Model file for the job. Use its own axes, mm. A direction names the side the tool comes from. Coordinates: 2 decimals unless noted, no trailing zeros. Order: outer loops, then holes, each group sorted by start corner. A loop starts at its lowest first (then second) coordinate and runs counter-clockwise, first axis right, second up. Notation, with made-up numbers: (-39, 80) -> (-12, 80) arc R30 cw to (-12, 119) -> close; hole circle Ø1 at (17.25, -19.75). An arc over 180 degrees is marked (long way). Return JSON: item names as keys, results as strings. Group by question number.
1) Cut at C-C (y = 46.5). Write the cut outline in (x, z), and give its area (3 significant figures).
2) Which spindle directions (+Z, -Z, +X, -X, +Y, -Y) get a long thin tool onto all of the face, cutting with end or side? Do faces 1 (the flat face through (15, 7, 13)), 2 (the flat face through (0, 35, 0)), 3 (the flat face through (11, 38, 0)), 4 (the flat face through (12.4, 10, -0.3)). Say none if no direction does.
3) Cut at D-D (y = 4). Write the cut outline in (x, z).
4) Pull direction Z, two halves, no side cores. Call faces 5 (the flat face through (-9, 7, -19)), 6 (the flat face through (-19, 5, 0)), 7 (the cylindrical face through (-8.895, 8.521, -17.615)), 8 (the cylindrical face through (-11.99, 25.84, -0.53)): +Z half, -Z half, draft (parallel to the pull), parting line (faces both ways), or undercut.
5) Cut at A-A (z = -16). Write the cut outline in (x, y).
6) Flat gauge pins, fed straight in: pin 1 (7 mm diameter, centred on y = 40, z = -2, fed in from +X); pin 2 (14 mm diameter, centred on x = -12, z = -16, fed in from +Y); pin 3 (19 mm diameter, centred on x = 12, z = 16, fed in from -Y); pin 4 (2 mm diameter, centred on y = 18, z = -10.5, fed in from +X). Where does each tip first touch, or does it go through?
7) Cut at B-B (z = 16). Write the cut outline in (x, y), and give its area (3 significant figures).
8) Probe line 1 (Z direction, x = -12, y = 8); line 2 (X direction, y = 6, z = 16); line 3 (Z direction, x = -12, y = 4.5). List the from-to ranges inside material, lowest first.
Autodesk Inventor part; units mm, degrees
ref_plane "YZ Plane" through (0, 0, 0) normal (1, 0, 0) x (0, 1, 0)
ref_plane "XZ Plane" through (0, 0, 0) normal (0, 1, 0) x (-1, 0, 0)
ref_plane "XY Plane" through (0, 0, 0) normal (0, 0, 1) x (1, 0, 0)
sketch "Эскиз1" plane through (0, 0, 0) normal (0, 0, 1) x (1, 0, 0)
  line L0 (-19, 10) -> (19, 10)
  line L1 (19, 10) -> (19, 0)
  line L2 (19, 0) -> (-19, 0)
  line L3 (-19, 0) -> (-19, 10)
  line L4 (12, 10) -> (12, 34)
  line L5 (12, 34) -> (11, 34)
  line L6 (11, 34) -> (11, 50)
  line L7 (11, 50) -> (4, 50)
  line L8 (4, 50) -> (4, 35)
  line L9 (4, 35) -> (0, 35)
  line L10 (0, 35) -> (0, 10)
  line L11 (12, 34) -> (12, 50)
  line L12 (12, 50) -> (11, 50)
  line L13 (4, 50) -> (-4, 50)
  line L14 (-4, 50) -> (-4, 35)
  line L15 (-4, 35) -> (0, 35)
  line L16 (-12, 34) -> (-11, 34)
  line L17 (-11, 34) -> (-11, 50)
  line L18 (-12, 34) -> (-12, 50)
  line L19 (-12, 50) -> (-11, 50)
  point P0 (0, 0)
  point P1 (0, 0)
  dimension "d0" = 38
  dimension "d1" = 50
  dimension "d2" = 40
  dimension "d3" = 16
  dimension "d4" = 15
  dimension "d5" = 22
  dimension "d6" = 4
  dimension "d7" = 24
  dimension "d13" = 8
extrude "Выдавливание1" add sketch "Эскиз1" along normal mid plane 46 contours L0 L1 L2 L3
revolve "Вращение1" add sketch "Эскиз1" angle 360 about axis through (0, 35, 0) along (0, -1, 0) contours L10 L9 L8 L7 L6 L5 L4 L0 | L5 L6 L12 L11
extrude "Выдавливание2" cut sketch "Эскиз1" along normal through all both and the other way through all contours L15 L14 L13 L8 L9 | L5 L6 L12 L11 | L18 L19 L17 L16
sketch "Эскиз2" plane through (-11, 34, 4.7958) normal (-1, 0, 0) x (0, 0, 1)
  arc A0 (-13.2958, 16) -> (3.7042, 16) centre (-4.7958, 16) ccw
  line L0 (-13.2958, 16) -> (3.7042, 16)
  line L1 (6.5179, 16) -> (-16.1095, 16)
  point P0 (-4.7958, 16)
  dimension "d16" = 8.5
extrude "Выдавливание4" cut sketch "Эскиз2" against normal through all
sketch "Эскиз3" plane through (-19, 0, 23) normal (0, -1, 0) x (1, 0, 0)
  point P0 (19, -23)
  point P1 (7, -7)
  point P2 (7, -39)
  point P3 (31, -7)
  dimension "d19" = 12
  dimension "d21" = 16
  dimension "d22" = 32
  dimension "d30" = 24
hole "Отверстие1" at (-12, 0, 16) direction (0, 1, 0) diameter 8 end through all
hole "Отверстие2" at (12, 0, 16) at (-12, 0, -16) direction (0, 1, 0) diameter 7 end through all counterbore diameter 12 counterbore depth 7
properties part number "Фиксатор"
Answers below:
{
 "1": {"outline": "(-9.17, -7.75) arc R12 ccw to (-4, -11.31) -> (-4, -7.75) -> close; (-9.17, 7.75) -> (-4, 7.75) -> (-4, 11.31) arc R12 ccw to start; (4, -11.31) arc R12 ccw to (9.17, -7.75) -> (4, -7.75) -> close; (4, 7.75) -> (9.17, 7.75) arc R12 ccw to (4, 11.31) -> close", "area": "43.9 mm^2"},
 "2": {"face 1": "-Y", "face 2": "+Z, -Z, +Y", "face 3": "+Z, -Z, +X, +Y", "face 4": "+Y"},
 "3": {"outline": "(-19, -23) -> (19, -23) -> (19, 23) -> (-19, 23) -> close; hole circle Ø12 at (-12, -16); hole circle Ø8 at (-12, 16); hole circle Ø12 at (12, 16)"},
 "4": {"face 5": "undercut", "face 6": "draft", "face 7": "undercut", "face 8": "parting line"},
 "5": {"outline": "(-19, 0) -> (-18, 0) -> (-18, 7) -> (-15.5, 7) -> (-15.5, 10) -> (-19, 10) -> close; (-8.5, 7) -> (-6, 7) -> (-6, 0) -> (19, 0) -> (19, 10) -> (-8.5, 10) -> close"},
 "6": {"pin 1": "stops at x = 11", "pin 2": "stops at y = 10", "pin 3": "stops at y = 0", "pin 4": "stops at x = 7.33"},
 "7": {"outline": "(-19, 0) -> (-16, 0) -> (-16, 10) -> (-19, 10) -> close; (-8, 0) -> (6, 0) -> (6, 7) -> (8.5, 7) -> (8.5, 10) -> (-8, 10) -> close; (15.5, 7) -> (18, 7) -> (18, 0) -> (19, 0) -> (19, 10) -> (15.5, 10) -> close", "area": "195 mm^2"},
 "8": {"line 1": "z = -23 to -19.5, -12.5 to 12, 20 to 23", "line 2": "x = -19 to -16, -8 to 6, 18 to 19", "line 3": "z = -23 to -22, -10 to 12, 20 to 23"}
}
